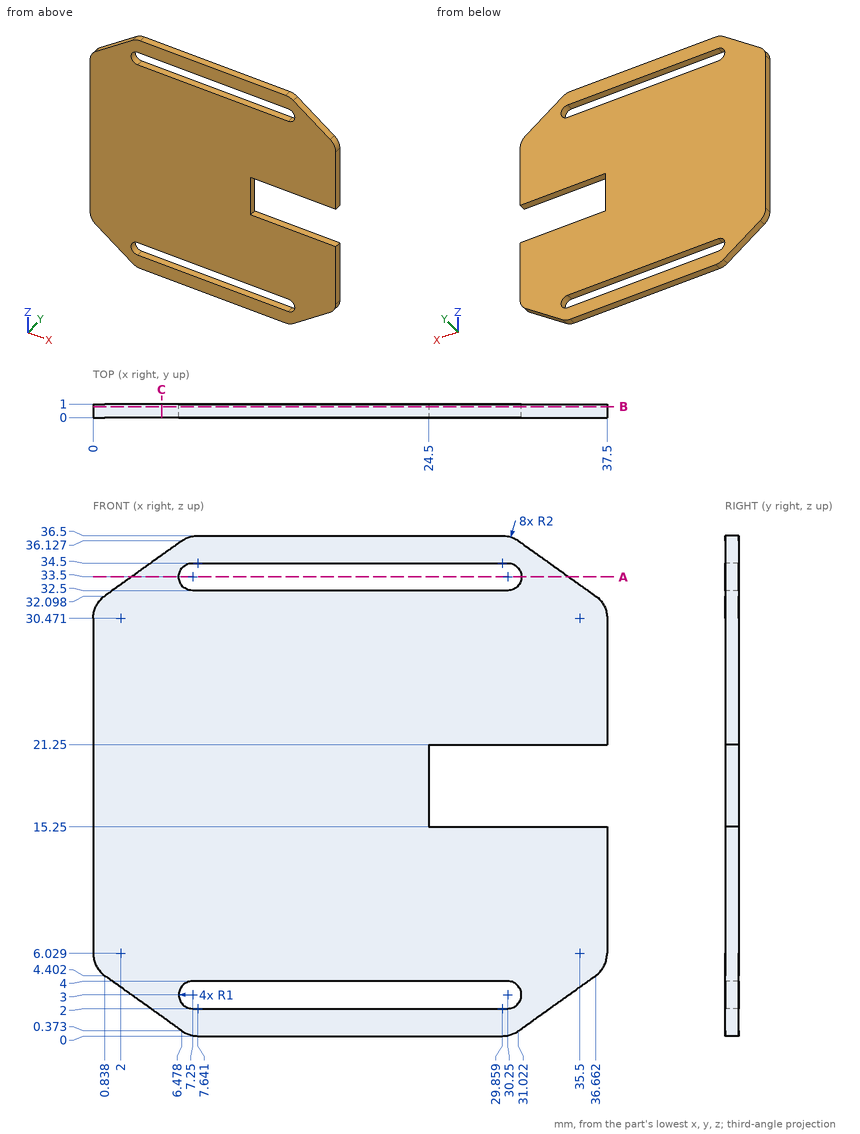
Can you work these out from the drawing? Everything is in mm from the part's minimum corner. Coordinates: 2 decimals unless noted, no trailing zeros. Loops run counter-clockwise (first coordinate to the right, second up) from the corner with the lowest first, then second, coordinate; pieces in that order, holes last.
1) I need wall thicknesses on probe 1 along Z at (x, y) = (20.5, 0.55); probe 2 along Z at (x, y) = (26, 0.6); probe 3 along Z at (x, y) = (7, 0.4) (1 decimal). Which ranges of each line are inside material? Lowest first, please.
2) Imagine slicing it at B-B on y = 0.8. List the corners of the cut face in (x, z) for me.
3) Imagine slicing it at C-C on x = 5. List the corners of the cut face in (y, z) for me.
4) Imagine slicing it at A-A on z = 33.5. List the corners of the cut face in (x, y) for me.
5) For pin 1 (6 mm diameter, centred on x = 15, z = 29.5, fed in from -Y), with a flat end and sliding along its axis, tell me the tip position at first contact or that it passes through.
Completed:
1. probe 1: z = 0 to 2, 4 to 32.5, 34.5 to 36.5
1. probe 2: z = 0 to 2, 4 to 15.25, 21.25 to 32.5, 34.5 to 36.5
1. probe 3: z = 0.1 to 2, 4 to 32.5, 34.5 to 36.4
2. outline: (0, 6.03) arc R2 ccw to (0.84, 4.4) - (6.48, 0.37) arc R2 ccw to (7.64, 0) - (29.86, 0) arc R2 ccw to (31.02, 0.37) - (36.66, 4.4) arc R2 ccw to (37.5, 6.03) - (37.5, 15.25) - (24.5, 15.25) - (24.5, 21.25) - (37.5, 21.25) - (37.5, 30.47) arc R2 ccw to (36.66, 32.1) - (31.02, 36.13) arc R2 ccw to (29.86, 36.5) - (7.64, 36.5) arc R2 ccw to (6.48, 36.13) - (0.84, 32.1) arc R2 ccw to (0, 30.47) - close; hole (7.25, 2) - (30.25, 2) arc R1 ccw to (30.25, 4) - (7.25, 4) arc R1 ccw to start; hole (7.25, 32.5) - (30.25, 32.5) arc R1 ccw to (30.25, 34.5) - (7.25, 34.5) arc R1 ccw to start
3. outline: (0, 1.43) - (1, 1.43) - (1, 35.07) - (0, 35.07) - close
4. outline: (2.8, 0) - (6.25, 0) - (6.25, 1) - (2.8, 1) - close; (31.25, 0) - (34.7, 0) - (34.7, 1) - (31.25, 1) - close
5. pin 1: stops at y = 0
